```python
from build123d import *

# Parameters (mm, degrees)
PAD019_DEPTH        = 5
SKETCH042_R         = 3
PAD023_DEPTH        = 4
FILLET018_R         = 1
SKETCH041_W         = 7
SKETCH041_H         = 5
PAD024_DEPTH        = 25
HOLE007_D           = 1.6
HOLE007_CBORE_D     = 3.7
HOLE007_CBORE_DEPTH = 1
POCKET018_DEPTH     = 5.001
POCKET019_DEPTH     = 10.001
FILLET019_R         = 1
FILLET020_R         = 0.5
FILLET021_R         = 1


with BuildPart() as part:
    # Sketch033 → Pad019 (new body, symmetric)
    with BuildSketch(Plane.YZ):
        Polygon((-5, 7.5), (-5, 10.5), (5, 10.5), (5, 7.5), (1.6, 7.5), (1.6, 6.5), (2, 6.5), (2, 4.5), (-2, 4.5), (-2, 6.5), (-1.6, 6.5), (-1.6, 7.5), align=None)
    extrude(amount=PAD019_DEPTH, both=True)

    # Sketch042 (on Face2 of Pad019) → Pad023 (join)
    with BuildSketch(Plane(origin=(0, 0, 10.5), x_dir=(0, -1, 0), z_dir=(0, 0, 1))):
        Circle(SKETCH042_R)
    extrude(amount=PAD023_DEPTH)

    # Fillet018
    fillet018_edges = [part.edges().sort_by_distance(p)[0] for p in [
        (0, 3, 10.5),
    ]]
    fillet(fillet018_edges, radius=FILLET018_R)

    # Sketch041 (on DatumPlane) → Pad024 (join)
    with BuildSketch(Plane(origin=(0, -5, 0), x_dir=(0, 0, -1), z_dir=(0, -1, 0))):
        with Locations((-11, 2.5)):
            Rectangle(SKETCH041_W, SKETCH041_H)
    extrude(amount=-PAD024_DEPTH)

    # Hole007 (through all)
    with Locations(Plane(origin=(0, 0, 14.5), x_dir=(0, -1, 0), z_dir=(0, 0, 1))):
        with Locations((0, 0)):
            CounterBoreHole(HOLE007_D / 2, HOLE007_CBORE_D / 2, HOLE007_CBORE_DEPTH)

    # Sketch044 (on DatumPlane) → Pocket018 (cut, through all)
    with BuildSketch(Plane(origin=(0, 0, 0), x_dir=(0, 1, 0), z_dir=(-1, 0, 0))):
        with BuildLine():
            ThreePointArc((7, -9.4), (5.4, -11), (7, -12.6))
            Line((7, -12.6), (16.5, -12.6))
            ThreePointArc((16.5, -12.6), (18.1, -11), (16.5, -9.4))
            Line((7, -9.4), (16.5, -9.4))
        make_face()
    extrude(amount=-POCKET018_DEPTH, mode=Mode.SUBTRACT)

    # Sketch034 → Pocket019 (cut, through all)
    with BuildSketch(Plane.YZ.offset(5)):
        Polygon((0.5, 8.3), (0.4, 4.3), (-0.4, 4.3), (-0.5, 8.3), (-4, 8.3), (-4, 9.1), (4, 9.1), (4, 8.3), align=None)
    extrude(amount=-POCKET019_DEPTH, mode=Mode.SUBTRACT)

    # Fillet019
    fillet019_edges = [part.edges().sort_by_distance(p)[0] for p in [
        (0, -5, 12.5),
        (2.5, -5, 14.5),
        (0, 11.5, 14.5),
        (0, -4, 14.5),
        (0, 20, 11),
        (0, 12.5, 7.5),
        (2.5, 20, 14.5),
        (2.5, 20, 7.5),
    ]]
    fillet(fillet019_edges, radius=FILLET019_R)

    # Fillet020
    fillet020_edges = [part.edges().sort_by_distance(p)[0] for p in [
        (-5, 0, 10.5),
        (-2.5, -5, 10.5),
        (0.5, -5, 10.5),
        (-5, -5, 9),
        (0, -5, 7.5),
        (-5, -3.3, 7.5),
        (-5, 3.3, 7.5),
        (-5, 5, 9),
        (-2.5, 5, 10.5),
        (-2.5, 5, 7.5),
        (0.5, 5, 7.5),
        (5, 20, 11),
        (5, 19.707107, 7.792893),
        (5, 10.3, 7.5),
        (5, -3.3, 7.5),
        (5, -5, 10.5),
        (5, -4.707107, 14.207107),
        (5, 7.5, 14.5),
        (5, 19.707107, 14.207107),
    ]]
    fillet(fillet020_edges, radius=FILLET020_R)

    # Fillet021
    fillet021_edges = [part.edges().sort_by_distance(p)[0] for p in [
        (0, -2, 4.5),
        (0, 2, 4.5),
    ]]
    fillet(fillet021_edges, radius=FILLET021_R)


with BuildPart() as part_1:
    # Body004 placement: moved
    add(part.part.moved(Location((-37.45, 0, 0))))


solid = part_1.part
```
Here's how the part is built. I have some questions about the finished solid (model axes, mm). A direction names the side the tool comes from. Coordinates: 2 decimals unless noted, no trailing zeros. Order: outer loops, then holes, each group sorted by start corner. A loop starts at its lowest first (then second) coordinate and runs counter-clockwise, first axis right, second up. Notation, with made-up numbers: (15, 32) -> (61, 32) arc R31 cw to (61, 68) -> close; hole circle Ø5 at (86, -10). An arc over 180 degrees is marked (long way). Return JSON: item names as keys, results as strings.
1) If we section it at B-B on z = 12.25: List the corners of the cut face in (x, y) for me.
Conclusion:
{"outline": "(-37.45, -4) arc R1 ccw to (-36.45, -5) -> (-32.95, -5) arc R0.5 ccw to (-32.45, -4.5) -> (-32.45, 6) -> (-37.45, 6) -> (-37.45, 3) arc R3 ccw to (-37.45, -3) -> close; (-37.45, 17.5) -> (-32.45, 17.5) -> (-32.45, 19.5) arc R0.5 ccw to (-32.95, 20) -> (-36.45, 20) arc R1 ccw to (-37.45, 19) -> close; hole circle Ø1.6 at (-37.45, 0)"}
2) If we section it at A-A on y = 7.25: List the corners of the cut face in (x, z) for me.
Conclusion:
{"outline": "(-37.45, 8.5) arc R1 ccw to (-36.45, 7.5) -> (-32.95, 7.5) arc R0.5 ccw to (-32.45, 8) -> (-32.45, 9.4) -> (-37.45, 9.4) -> close; (-37.45, 12.6) -> (-32.45, 12.6) -> (-32.45, 14) arc R0.5 ccw to (-32.95, 14.5) -> (-36.45, 14.5) arc R1 ccw to (-37.45, 13.5) -> close"}
3) Thinking about a two-plate mould opening in Z: for faces 1 (the cylindrical face through (-37.52, -1.699, 4.785)), 2 (the flat face through (-35, 7, 14.5)), 3 (the flat face through (-37, 2, 8.3)), which applies, +Z half, -Z half, draft (parallel to the pull), parting line (faces both ways), or undercut?
Conclusion:
{"face 1": "-Z half", "face 2": "+Z half", "face 3": "undercut"}
4) I'm going to push flat-ended pins straight in: P1, Ø1.1, axis at x = -36.5, z = 6, coming from the -Y side; P2, Ø0.9, axis at x = -38, y = -3, coming from the -Z side; P3, Ø3, axis at x = -37.5, y = 0, coming from the +Z side. Where does each tip first touch, or does it pass through?
Conclusion:
{"P1": "stops at y = -2", "P2": "stops at z = 7.5", "P3": "stops at z = 13.5"}
5) If we section it at D-D on z = 11: List the corners of the cut face in (x, y) for me.
Conclusion:
{"outline": "(-37.45, -4) arc R1 ccw to (-36.45, -5) -> (-32.95, -5) arc R0.5 ccw to (-32.45, -4.5) -> (-32.45, 5.4) -> (-37.45, 5.4) -> (-37.45, 3.13) arc R3.13 ccw to (-37.45, -3.13) -> close; (-37.45, 18.1) -> (-32.45, 18.1) -> (-32.45, 19.5) arc R0.5 ccw to (-32.95, 20) -> (-36.45, 20) arc R1 ccw to (-37.45, 19) -> close; hole circle Ø1.6 at (-37.45, 0)"}
6) On a 3-axis mill with a long thin cutter (end or side, diameter ignored), from which of +Z, -Z, +X, -X, +Y, -Y can I reach the whole of each face in a straight line? I mean faces 4 (the flat face through (-41.7, -0.1, 10.5)), 5 (the flat face through (-37, -2, 8.3)), 6 (the cylindrical face through (-37.4, -0.8, 6.4)). Say none if no direction works.
Conclusion:
{"face 4": "+Z, -X", "face 5": "+X, -X", "face 6": "+Z, -Z"}
7) If I drill on probe 1 along Z at (x, y) = (-41.5, -2.25); probe 2 along Z at (x, y) = (-36, 11); probe 3 along X at (y, z) = (0, 13.9), over which ranges is the centre line in solid material (lowest first)?
Conclusion:
{"probe 1": "z = 7.5 to 8.3, 9.1 to 10.5", "probe 2": "z = 7.5 to 9.4, 12.6 to 14.5", "probe 3": "x = -40.45 to -39.3, -35.6 to -32.45"}
8) If we section it at C-C on y = 0: List the corners of the cut face in (x, z) for me, plus the area to 3 significant figures.
Conclusion:
{"outline": "(-42.45, 9.1) -> (-38.25, 9.1) -> (-38.25, 13.5) -> (-39.3, 13.5) -> (-39.3, 14.5) -> (-40.45, 14.5) -> (-40.45, 11.5) arc R1 cw to (-41.45, 10.5) -> (-41.95, 10.5) arc R0.5 ccw to (-42.45, 10) -> close; (-36.65, 9.1) -> (-32.45, 9.1) -> (-32.45, 14) arc R0.5 ccw to (-32.95, 14.5) -> (-35.6, 14.5) -> (-35.6, 13.5) -> (-36.65, 13.5) -> close", "area": "35.4 mm²"}
